Design review of the part shown in the three views and the two pictorial views. Dimensions are in mm from the part's minimum x, y and z. A direction names the side the tool comes from. Give positions to 0.01 mm unless a question says otherwise; leave off trailing zeros. Loops run counter-clockwise (first coordinate to the right, second up) from the corner with the lowest first, then second, coordinate; pieces in that order, holes last. Notation, with made-up numbers: (-35.5, 30) - (16.5, 30) arc R38 ccw to (16.5, 68) - close; hole circle Ø2 at (48.25, -24). An arc over 180 degrees is marked (long way). Use CSV: the item, a comma, the result in double quotes. Start each with the question number.
1. Take a section at B-B on x = 40.5. Give the boundary of the cut face in (y, z).
2. Take a section at A-A on z = 91. Give the boundary of the cut face in (x, y).
3. Wall thickness on line 1 (Y direction, x = 30, z = 92); line 2 (X direction, y = 5, z = 27): over which ranges is each line inside the solid? List them lowest first.
4. For the marked faces 1 and 2, list the 3-axis set-ups (+Z, -Z, +X, -X, +Y, -Y) from which the entire face can be reached by the end or side of a thin tool; tool diameter is ignored.
5. For pin 1 (1 mm diameter, centred on y = 40, z = 24.5, fed in from -X); pin 2 (17 mm diameter, centred on x = 24.5, z = 36.5, fed in from +Y), all flat-tipped, find the tip position at first contact; note any pin that passes through.
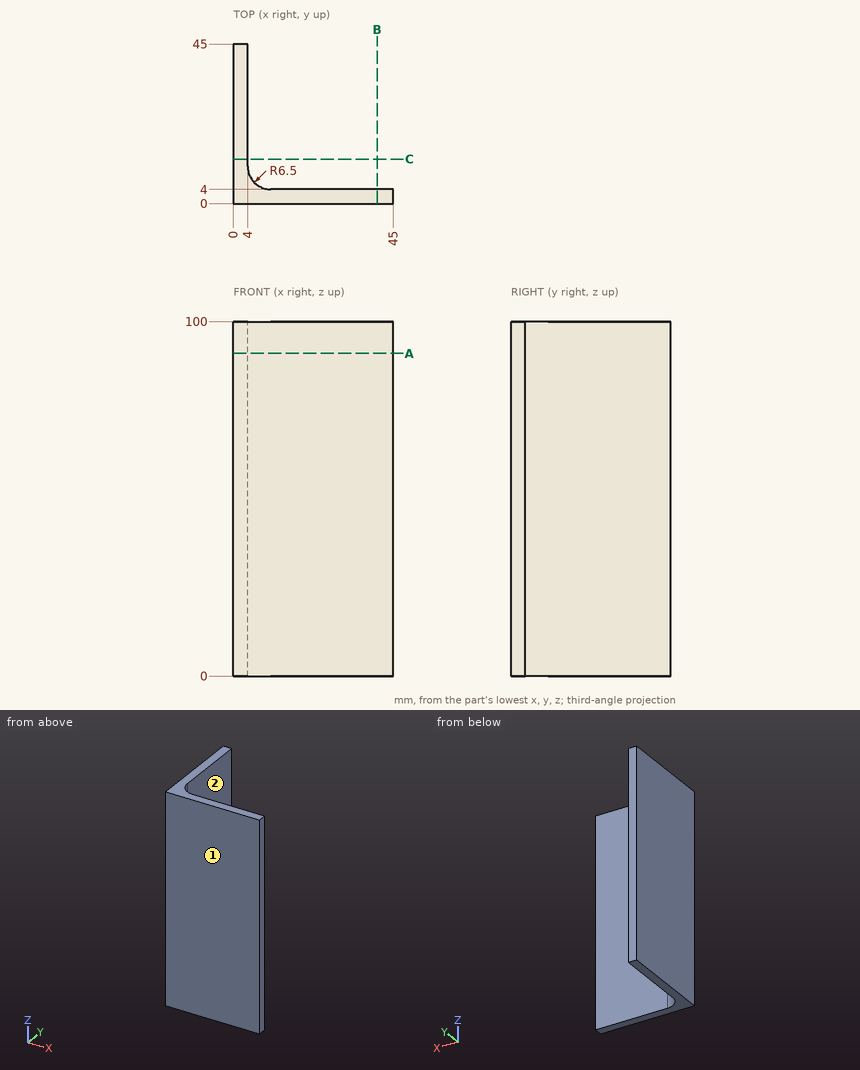
Check result:
1,outline,"(0, 0) - (4, 0) - (4, 100) - (0, 100) - close"
2,outline,"(0, 0) - (45, 0) - (45, 4) - (10.5, 4) arc R6.5 cw to (4, 10.5) - (4, 45) - (0, 45) - close"
3,line 1,"y = 0 to 4"
3,line 2,"x = 0 to 7.04"
4,face 1,"+Z, -Z, +X, -X, -Y"
4,face 2,"+Z, -Z, +X, +Y"
5,pin 1,"stops at x = 0"
5,pin 2,"stops at y = 4"
